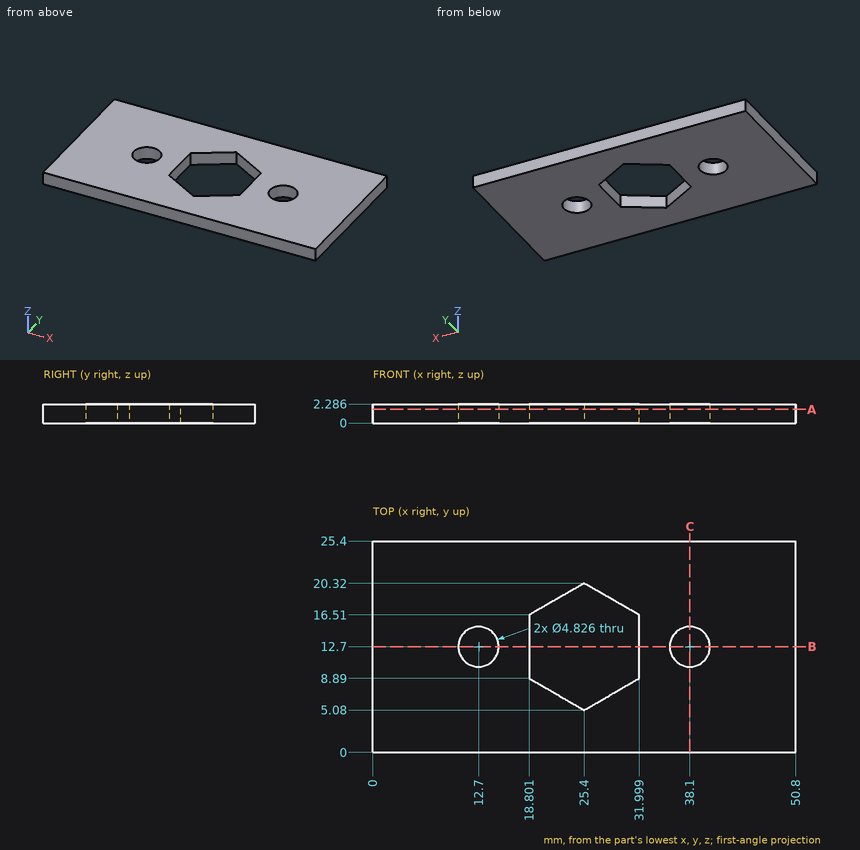
Here's the drawing with two shaded views (mm, measured from the low corner). I have some questions. Give positions to 0.01 mm unless a question says otherwise; leave off trailing zeros. Order: outer loops, then holes, each group sorted by start corner. A loop starts at its lowest first (then second) coordinate and runs counter-clockwise, first axis right, second up.
Q1. Suppose I cut it at C-C, the plane x = 38.1. Write out the boundary of the cut face in (y, z), and give its area (3 significant figures).
Q2. If I drill on line 1 along X through (y, z) = (12, 0.45); line 2 along X through (y, z) = (14, 0.15); line 3 along Y through (x, z) = (12.7, 0.6), over which ranges is the centre line in solid material (lowest first)?
Q3. I'm going to push a flat-ended pin straight in: P1, Ø5.5, axis at x = 38.1, y = 12.7, coming from the -Z side. Where does the tip first touch, or does it pass through?
Q4. Suppose I cut it at A-A, the plane z = 1.65. Write out the boundary of the cut face in (x, y), and give its area (3 significant figures).
Q5. Suppose I cut it at B-B, the plane y = 12.7. Write out the boundary of the cut face in (x, z).
Solution:
1. outline: (0, 0) - (10.29, 0) - (10.29, 2.29) - (0, 2.29) - close; (15.11, 0) - (25.4, 0) - (25.4, 2.29) - (15.11, 2.29) - close
1. area: 47.0 mm2
2. line 1: x = 0 to 10.39, 15.01 to 18.8, 32 to 35.79, 40.41 to 50.8
2. line 2: x = 0 to 10.67, 14.73 to 18.8, 32 to 36.07, 40.13 to 50.8
2. line 3: y = 0 to 10.29, 15.11 to 25.4
3. P1: stops at z = 0
4. outline: (0, 0) - (50.8, 0) - (50.8, 25.4) - (0, 25.4) - close; hole circle Ø4.83 at (12.7, 12.7); hole (18.8, 8.89) - (25.4, 5.08) - (32, 8.89) - (32, 16.51) - (25.4, 20.32) - (18.8, 16.51) - close; hole circle Ø4.83 at (38.1, 12.7)
4. area: 1,100 mm2
5. outline: (0, 0) - (10.29, 0) - (10.29, 2.29) - (0, 2.29) - close; (15.11, 0) - (18.8, 0) - (18.8, 2.29) - (15.11, 2.29) - close; (32, 0) - (35.69, 0) - (35.69, 2.29) - (32, 2.29) - close; (40.51, 0) - (50.8, 0) - (50.8, 2.29) - (40.51, 2.29) - close
